Model file for the job. Use its own axes, mm. A direction names the side the tool comes from. Give positions to 0.01 mm unless a question says otherwise; leave off trailing zeros. Loops run counter-clockwise (first coordinate to the right, second up) from the corner with the lowest first, then second, coordinate; pieces in that order, holes last. Notation, with made-up numbers: M -16,-32.75 L 8,-32.75 A10 ccw 8,-21.75 Z; hole C 9,77 d4. An arc over 180 degrees is marked long. Answer in a Markdown table with one row per item.
```python
from build123d import *

# Parameters (mm, degrees)
F7_R     = 13.2729716618
F8_DEPTH = 29.2


with BuildPart() as f3:
    # F0 (on Front) → F3 section 0
    with BuildSketch(Plane.XZ, mode=Mode.PRIVATE) as f3_s0:
        Polygon((-27.3326151073, 0), (-34.8543561995, -34.8543561995), (0, -27.3326151073), (34.8543561995, -34.8543561995), (27.3326151073, 0), (34.8543561995, 34.8543561995), (0, 27.3326151073), (-34.8543561995, 34.8543561995), align=None)
    loft([f3_s0.sketch, Vertex(-2.2883485071, -18.5, 0)])

    # F3_face (on face) → F6 section 0
    with BuildSketch(Plane(origin=(0, 0, 0), x_dir=(-1, 0, 0), z_dir=(0, 1, 0)), mode=Mode.PRIVATE) as f6_s0:
        Polygon((27.3326151073, 0), (34.8543561995, 34.8543561995), (0, 27.3326151073), (-34.8543561995, 34.8543561995), (-27.3326151073, 0), (-34.8543561995, -34.8543561995), (0, -27.3326151073), (34.8543561995, -34.8543561995), align=None)
    loft([f6_s0.sketch, Vertex(0, 18.5, 0)])

    # F7 (on Front) → F8 (cut, symmetric)
    with BuildSketch(Plane.XZ):
        Circle(F7_R)
    extrude(amount=F8_DEPTH, both=True, mode=Mode.SUBTRACT)


solid = f3.part
```
Q1. Mould opens along X. For faces 1 (the face through (-14.441, -5.542, -22.113)), 2 (the face through (-22.764, -5.542, 13.594)), 3 (the face through (21.88, -5.19, 13.23)) say: released by +X, released by -X, zero draft, split by the parting line, or undercut.
Reported:
| item | result |
|---|---|
| face 1 | undercut |
| face 2 | released by -X |
| face 3 | released by +X |
Q2. Saw through at B-B (y = -6.5). Give the cut face in (x, z), and give its area (3 significant figures).
Reported:
| item | result |
|---|---|
| outline | M -23.41,-22.61 L -0.8,-17.73 L 21.8,-22.61 L 16.93,0 L 21.8,22.61 L -0.8,17.73 L -23.41,22.61 L -18.53,0 Z; hole C 0,0 d26.55 |
| area | 1,050 mm² |
Q3. Saw through at D-D (x = 2). Give the cut face in (y, z), and give its area (3 significant figures).
Reported:
| item | result |
|---|---|
| outline | M -10.09,-13.12 L 0,-27.76 L 9.91,-13.12 Z; M -10.09,13.12 L 9.91,13.12 L 0,27.76 Z |
| area | 293 mm² |
Q4. Probe probe 1 along X at (y, z) = (-3, 0); probe 2 along X at (y, z) = (-3.5, 6); probe 3 along Z at (x, y) = (0, -5.5). List the from-to ranges inside material, lowest first.
Reported:
| item | result |
|---|---|
| probe 1 | -23.27 to -13.27, 13.27 to 22.53 |
| probe 2 | -23.89 to -11.84, 11.84 to 23.02 |
| probe 3 | -19.35 to -13.27, 13.27 to 19.35 |
Q5. 3-axis set-ups, long thin cutter, end or side, ignore diameter. For faces 4 (the face through (12.37, -5.19, -22.47)), 5 (the face through (21.99, -5.19, -13.76)), 6 (the face through (13.149, 5.352, 22.263)): which of +Z, -Z, +X, -X, +Y, -Y reach the whole face in a straight line?
Reported:
| item | result |
|---|---|
| face 4 | -Z, -Y |
| face 5 | +X, -Y |
| face 6 | +Z, +Y |
Q6. Saw through at C-C (z = 22). Give the cut face in (x, y).
Reported:
| item | result |
|---|---|
| outline | M -32.08,0 L -22.84,-6.82 L -0.45,-3.61 L 21.16,-6.82 L 32.08,0 L 22,6.82 L 0,3.61 L -22,6.82 Z |
Q7. Drop flat-ended pins along their axis: pin 1 (5 mm diameter, centred on x = 14, z = -17.5, fed in from +Y); pin 2 (1.5 mm diameter, centred on x = 8, y = -3.5, fed in from -Z); pin 3 (1.5 mm diameter, centred on x = -19, z = 4.5, fed in from -Y); pin 4 (1.5 mm diameter, centred on x = 21, y = 10, fed in from +Z). Give the stop position or say it passes through.
Reported:
| item | result |
|---|---|
| pin 1 | y = 10.43 |
| pin 2 | z = -25.08 |
| pin 3 | y = -7.44 |
| pin 4 | through |
Q8. Saw through at A-A (x = -29). Give the cut face in (y, z).
Reported:
| item | result |
|---|---|
| outline | M -3.33,-28.59 L 0,-33.59 L 3.11,-29 L 0,-7.73 Z; M -3.33,28.59 L 0,7.73 L 3.11,29 L 0,33.59 Z |
